from build123d import *

# Parameters (mm, degrees)
SKETCH1_W                                       = 38.1
SKETCH1_H                                       = 25.4
BOSS_EXTRUDE1_DEPTH                             = 6.35
SKETCH6_R                                       = 9.128125
CUT_EXTRUDE1_DEPTH                              = 24.759524406
SKETCH8_W                                       = 14.2875
SKETCH8_H                                       = 25.4
CUT_EXTRUDE2_DEPTH                              = 2.38125
SKETCH14_W                                      = 38.1
SKETCH14_H                                      = 25.4
SKETCH14_R                                      = 11.3665
CUT_EXTRUDE3_DEPTH                              = 1.190625
SKETCH19_R                                      = 10.0965
CUT_EXTRUDE4_DEPTH                              = 2.38125
F_2_CLEARANCE_HOLE1_D                           = 2.4384
CBORE_FOR_2_PAN_HEAD_MACHINE_SCREW1_D           = 2.4384
CBORE_FOR_2_PAN_HEAD_MACHINE_SCREW1_CBORE_D     = 4.7625
CBORE_FOR_2_PAN_HEAD_MACHINE_SCREW1_CBORE_DEPTH = 2.38125


with BuildPart() as part:
    # Sketch1 → Boss-Extrude1 (new body)
    with BuildSketch(Plane.XY):
        Rectangle(SKETCH1_W, SKETCH1_H)
    extrude(amount=BOSS_EXTRUDE1_DEPTH)

    # Sketch6 → Cut-Extrude1 (cut, through all)
    with BuildSketch(Plane.XY.offset(6.35)):
        Circle(SKETCH6_R)
    extrude(amount=-CUT_EXTRUDE1_DEPTH, mode=Mode.SUBTRACT)

    # Sketch8 → Cut-Extrude2 (cut)
    with BuildSketch(Plane.XY.offset(6.35)):
        Rectangle(SKETCH8_W, SKETCH8_H)
    extrude(amount=-CUT_EXTRUDE2_DEPTH, mode=Mode.SUBTRACT)

    # Sketch14 → Cut-Extrude3 (cut)
    with BuildSketch(Plane(origin=(0, 0, 0), x_dir=(-1, 0, 0), z_dir=(0, 0, -1))):
        Rectangle(SKETCH14_W, SKETCH14_H)
        Circle(SKETCH14_R, mode=Mode.SUBTRACT)
    extrude(amount=-CUT_EXTRUDE3_DEPTH, mode=Mode.SUBTRACT)

    # Sketch19 → Cut-Extrude4 (cut)
    with BuildSketch(Plane(origin=(0, 0, 0), x_dir=(-1, 0, 0), z_dir=(0, 0, -1))):
        Circle(SKETCH19_R)
    extrude(amount=-CUT_EXTRUDE4_DEPTH, mode=Mode.SUBTRACT)

    # #2 Clearance Hole1 (through all)
    with Locations(Plane(origin=(0, 0, 1.190625), x_dir=(-1, 0, 0), z_dir=(0, 0, -1))):
        with Locations((-9.779, 9.779), (9.779, 9.779), (9.779, -9.779), (-9.779, -9.779)):
            Hole(F_2_CLEARANCE_HOLE1_D / 2)

    # CBORE for #2 Pan Head Machine Screw1 (through all)
    with Locations(Plane(origin=(0, 0, 1.190625), x_dir=(-1, 0, 0), z_dir=(0, 0, -1))):
        with Locations((-15.875, 7.9375), (-15.875, -7.9375), (15.875, -7.9375), (15.875, 7.9375)):
            CounterBoreHole(CBORE_FOR_2_PAN_HEAD_MACHINE_SCREW1_D / 2, CBORE_FOR_2_PAN_HEAD_MACHINE_SCREW1_CBORE_D / 2, CBORE_FOR_2_PAN_HEAD_MACHINE_SCREW1_CBORE_DEPTH)


solid = part.part
Read the model definition and answer for the solid it produces. Units are mm, in the model's axes. A direction names the side the tool comes from. Give positions to 0.01 mm unless a question says otherwise; leave off trailing zeros. Loops run counter-clockwise (first coordinate to the right, second up) from the corner with the lowest first, then second, coordinate; pieces in that order, holes last. Notation, with made-up numbers: (65.5, 17.5) - (107.5, 17.5) arc R28 cw to (107.5, 48.5) - close; hole circle Ø1 at (45.25, 49.25). An arc over 180 degrees is marked (long way). Answer as CSV lines item,"result". Start each with the question number.
1) Each of these flat-tipped pins is pushed along its axis until it touches: pin 1 Ø3 at (x, y) = (-15.88, -7.94) entering from -Z; pin 2 Ø2 at (x, y) = (-12.5, 3.5) entering from -Z; pin 3 Ø14.5 at (x, y) = (0, 0) entering from -Z; pin 4 Ø7.5 at (x, y) = (-1.5, 10) entering from +Z. Where does it stop, or does it pass through?
2) Find section C-C (z = 4.75). State how many separate pieces and enclosed holes the cut face has, then the cut area to 3 significant figures.
3) Determine the mould class of faces 1 (the face through (13, 0, 6.35)), 2 (the face through (-0.3, 12.7, 3.7)), 3 (the face through (-9.216, -10.861, 3.806)) for opening direction Y: released by +Y, released by -Y, zero draft, split by the parting line, or undercut.
4) Which of the six approach directions +Z, -Z, +X, -X, +Y, -Y give full straight-line access (tool end or side, diameter ignored) to faces 4 (the face through (-17, -9, 3.572)), 5 (the face through (7.144, 9, 5)), 6 (the face through (14.657, -7.884, 4.98))?
5) Find section A-A (x = 0). Write down the section's boundary in (y, z).
6) Find section B-B (y = 0). Write down the section's boundary in (x, z).
7) Straight lines are drawn through the part: L1, parallel to Y at x = -10.5, z = 4; L2, parallel to Y at x = -15.5, z = 3.75; L3, parallel to X at y = -6.5, z = 4.5. For each, find the intervals that lie inside material, in ascending order. Write a range as from..to.
8) Find section D-D (x = 12). Write down the section's boundary in (y, z).
Findings below:
1,pin 1,"z = 3.57"
1,pin 2,"z = 1.19"
1,pin 3,"through"
1,pin 4,"z = 3.97"
2,separate pieces,"2"
2,enclosed holes,"8"
2,area,"537 mm^2"
3,face 1,"zero draft"
3,face 2,"released by +Y"
3,face 3,"undercut"
4,face 4,"-Z"
4,face 5,"+Z, +Y, -Y"
4,face 6,"+Z, -Z"
5,outline,"(-12.7, 1.19) - (-11.37, 1.19) - (-11.37, 0) - (-10.1, 0) - (-10.1, 2.38) - (-9.13, 2.38) - (-9.13, 3.97) - (-12.7, 3.97) - close; (9.13, 2.38) - (10.1, 2.38) - (10.1, 0) - (11.37, 0) - (11.37, 1.19) - (12.7, 1.19) - (12.7, 3.97) - (9.13, 3.97) - close"
6,outline,"(-19.05, 1.19) - (-11.37, 1.19) - (-11.37, 0) - (-10.1, 0) - (-10.1, 2.38) - (-9.13, 2.38) - (-9.13, 6.35) - (-19.05, 6.35) - close; (9.13, 2.38) - (10.1, 2.38) - (10.1, 0) - (11.37, 0) - (11.37, 1.19) - (19.05, 1.19) - (19.05, 6.35) - (9.13, 6.35) - close"
7,L1,"-12.7..-10.76, -8.8..8.8, 10.76..12.7"
7,L2,"-12.7..-9.1, -6.78..6.78, 9.1..12.7"
7,L3,"-19.05..-7.14, 7.14..19.05"
8,outline,"(-12.7, 1.19) - (12.7, 1.19) - (12.7, 6.35) - (-12.7, 6.35) - close"
